Here's how the part is built. I have some questions about the finished solid (model axes, mm). A direction names the side the tool comes from. Round coordinates to 2 decimals unless told otherwise and drop trailing zeros. Loops run counter-clockwise (first coordinate to the right, second up) from the corner with the lowest first, then second, coordinate; pieces in that order, holes last. Notation, with made-up numbers: M 81,67 L 138,67 A20 cw 138,99 Z; hole C 22.25,59.5 d4. An arc over 180 degrees is marked long. Answer as a JSON object with one key per item and string values.
from build123d import *

# Parameters (mm, degrees)
SKETCH1_W           = 10.11
SKETCH1_H           = 2
EXTRUDE_THIN1_DEPTH = 8
CHAMFER1_SIZE       = 8
SKETCH2_R           = 3.15
BOSS_EXTRUDE1_DEPTH = 2
SKETCH6_R           = 8.5
SKETCH6_R_2         = 4.25
BOSS_EXTRUDE4_DEPTH = 2
FILLET4_R           = 2


with BuildPart() as part:
    # Sketch1 → Extrude-Thin1 (new body)
    with BuildSketch(Plane(origin=(0, 0, 0), x_dir=(0, 0, -1), z_dir=(1, 0, 0))):
        with Locations((-5.055, 0)):
            Rectangle(SKETCH1_W, SKETCH1_H)
    extrude(amount=EXTRUDE_THIN1_DEPTH)

    # Chamfer1
    chamfer1_edges = [part.edges().sort_by_distance(p)[0] for p in [
        (0, 0, 10.11),
    ]]
    chamfer(chamfer1_edges, length=CHAMFER1_SIZE - 0.0001)  # a hair under: the kernel refuses the full size

    # Sketch2 → Boss-Extrude1 (add)
    with BuildSketch(Plane(origin=(0, 1, 0), x_dir=(1, 0, 0), z_dir=(0, 1, 0))):
        with BuildLine():
            Line((0, -0.43455532), (0, 0))
            ThreePointArc((0, 0), (4.444005662, 0.947416312), (8.29515392, 3.358938877))
            ThreePointArc((8.29515392, 3.358938877), (12.175107047, -2.736751195), (19, -5.11))
            Line((19, -5.11), (30, -5.11))
            ThreePointArc((30, -5.11), (35, -10.11), (30, -15.11))
            Line((30, -15.11), (19, -15.11))
            ThreePointArc((19, -15.11), (9.319017932, -12.745412155), (1.818181818, -6.184151066))
            ThreePointArc((1.818181818, -6.184151066), (0.465374108, -3.449668766), (0, -0.43455532))
        make_face()
        with Locations(Location((30, -10.11, 0), (0, 0, 270))):
            Circle(SKETCH2_R, mode=Mode.SUBTRACT)
        with Locations(Location((19, -10.11, 0), (0, 0, 90))):
            Circle(SKETCH2_R, mode=Mode.SUBTRACT)
    extrude(amount=-BOSS_EXTRUDE1_DEPTH)

    # Sketch6 → Boss-Extrude4 (add)
    with BuildSketch(Plane.XZ.offset(1)):
        with Locations((4, -7.5)):
            Circle(SKETCH6_R)
        with Locations(Location((4, -7.5, 0), (0, 0, 270))):
            Circle(SKETCH6_R_2, mode=Mode.SUBTRACT)
    extrude(amount=-BOSS_EXTRUDE4_DEPTH)

    # Fillet4
    fillet4_edges = [part.edges().sort_by_distance(p)[0] for p in [
        (0, 0, 0),
        (9.243332379, 0, -0.809897941),
    ]]
    fillet(fillet4_edges, radius=FILLET4_R)


solid = part.part
Item 1: I want a section at D-D, the plane y = -0.5. State how many separate pieces and enclosed holes the cut face has, then the cut area to 3 significant figures.
Resolved:
{"separate pieces": "1", "enclosed holes": "3", "area": "441 mm²"}
Item 2: Please list where these lines run through material, in increasing order: probe 1 along Z at (x, y) = (19, 0.15); probe 2 along X at (y, z) = (0.6, -7.5); probe 3 along X at (y, z) = (0.95, 11.5). Write a range as from..to.
Resolved:
{"probe 1": "5.11..6.96, 13.26..15.11", "probe 2": "-4.5..-0.25, 8.25..12.5", "probe 3": "7.23..16.17, 21.83..27.17, 32.83..34.8"}
Item 3: I want a section at C-C, the plane z = 8. Please give me the cut outline in (x, y), then the cut area to 3 significant figures.
Resolved:
{"outline": "M 3.25,-1 L 16.66,-1 L 16.66,1 L 3.25,1 Z; M 21.34,-1 L 27.66,-1 L 27.66,1 L 21.34,1 Z; M 32.34,-1 L 34.53,-1 L 34.53,1 L 32.34,1 Z", "area": "43.9 mm²"}
Item 4: On a 3-axis mill with a long thin cutter (end or side, diameter ignored), from which of +Z, -Z, +X, -X, +Y, -Y can I reach the whole of each face in a straight line? I mean faces 1 (the face through (24, 0, 5.11)), 2 (the face through (11, -1, 3)), 3 (the face through (0, 0, 1.6)). Say none if no direction works.
Resolved:
{"face 1": "-Z, +X, +Y, -Y", "face 2": "+Z, -Z, +X, -X, -Y", "face 3": "+Z, -X, +Y, -Y"}
Item 5: I'm going to push flat-ended pins straight in: pin 1 Ø5 at (x, z) = (28.5, 2.5) entering from -Y; pin 2 Ø1 at (y, z) = (-1, -7) entering from +X; pin 3 Ø1 at (x, y) = (28, -1) entering from -Z. Where does each tip first touch, or does it pass through?
Resolved:
{"pin 1": "through", "pin 2": "x = 12.5", "pin 3": "z = 5.11"}
Item 6: If we mould it in two halves opening along Z, with no side actions, what happens to faces 4 (the face through (25, 0, 15.11)), 5 (the face through (26.925, 0.014, 9.427)), 6 (the face through (14.02, 0.01, 3.92)), 7 (the face through (35, 0, 10))? For each: pulls with the +Z half, pulls with the -Z half, needs draft (parallel to the pull), parting line crosses it, or undercut.
Resolved:
{"face 4": "pulls with the +Z half", "face 5": "undercut", "face 6": "undercut", "face 7": "parting line crosses it"}
Item 7: I want a section at A-A, the plane z = -7.5. Please give me the cut outline in (x, y).
Resolved:
{"outline": "M -4.5,-1 L -0.25,-1 L -0.25,1 L -4.5,1 Z; M 8.25,-1 L 12.5,-1 L 12.5,1 L 8.25,1 Z"}
Item 8: I want a section at B-B, the plane x = 11. Please give me the cut outline in (y, z).
Resolved:
{"outline": "M -1,-12.32 L 1,-12.32 L 1,-2.68 L -1,-2.68 Z; M -1,1.66 L 1,1.66 L 1,13.53 L -1,13.53 Z"}
